The drawing under review shows one solid part. Ordinate dimensions are in mm from its lowest x, y, z. Give positions to 0.01 mm unless a question says otherwise; leave off trailing zeros. Order: outer loops, then holes, each group sorted by start corner. A loop starts at its lowest first (then second) coordinate and runs counter-clockwise, first axis right, second up. Notation, with made-up numbers: (68, -7) - (92, -7) arc R14 cw to (92, 6) - close; hole circle Ø5 at (88.5, -38). An arc over 180 degrees is marked (long way). Answer as a JSON object with one key per item and string values. Group by question number.
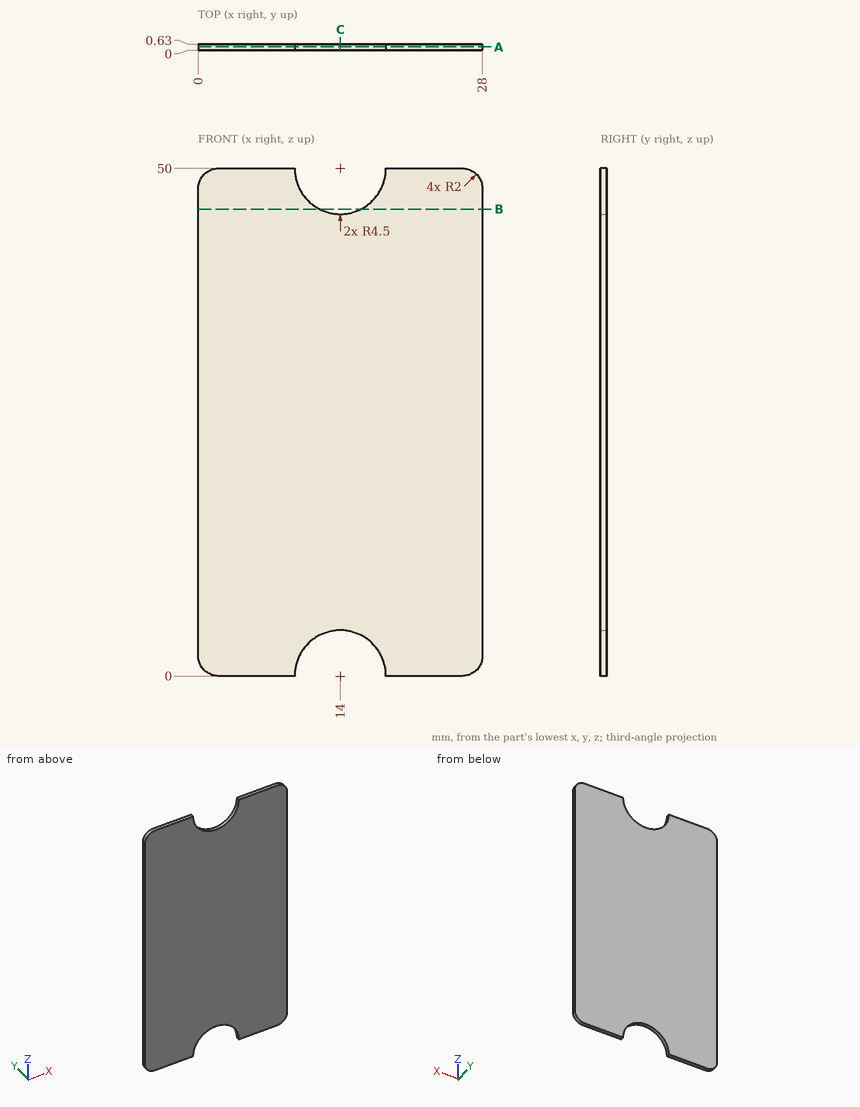
1) For line 1 (X direction, y = 0.15, z = 47); line 2 (Z direction, x = 1.5, y = 0.3); line 3 (Z direction, x = 14.75, y = 0.2), list the stretches that pass through material, from the lowest coordinate up.
2) Consider section B-B (z = 46). Give the boundary of the cut face in (x, y).
3) For pin 1 (10 mm diameter, centred on x = 14.5, z = 21.5, fed in from -Y), flat-tipped, find the tip position at first contact; note if it passes through.
4) Consider section A-A (y = 0.35). Give the boundary of the cut face in (x, z), plus the area to 3 significant figures.
5) Consider section C-C (x = 14). Give the boundary of the cut face in (y, z).
Result set:
{
 "1": {"line 1": "x = 0 to 10.65, 17.35 to 28", "line 2": "z = 0.06 to 49.94", "line 3": "z = 4.44 to 45.56"},
 "2": {"outline": "(0, 0) - (11.94, 0) - (11.94, 0.63) - (0, 0.63) - close; (16.06, 0) - (28, 0) - (28, 0.63) - (16.06, 0.63) - close"},
 "3": {"pin 1": "stops at y = 0"},
 "4": {"outline": "(0, 2) arc R2 ccw to (2, 0) - (9.5, 0) arc R4.5 cw to (18.5, 0) - (26, 0) arc R2 ccw to (28, 2) - (28, 48) arc R2 ccw to (26, 50) - (18.5, 50) arc R4.5 cw to (9.5, 50) - (2, 50) arc R2 ccw to (0, 48) - close", "area": "1,330 mm2"},
 "5": {"outline": "(0, 4.5) - (0.63, 4.5) - (0.63, 45.5) - (0, 45.5) - close"}
}
